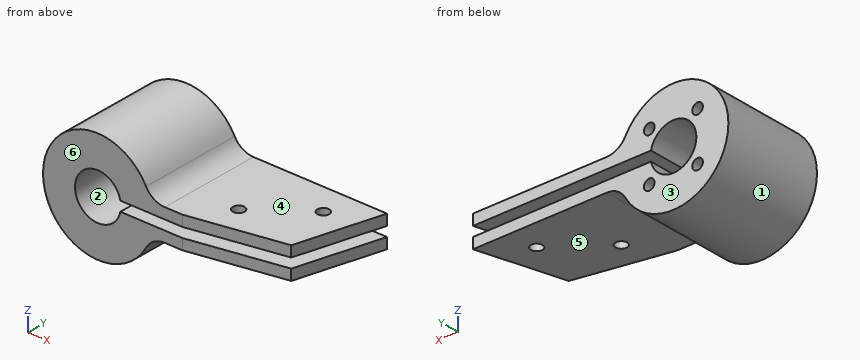
from build123d import *

# Parameters (mm, degrees)
BOSS_EXTRUDE1_DEPTH = 48
FILLET1_R           = 10
SKETCH5_R           = 2.5
CUT_EXTRUDE3_DEPTH  = 10
BOSS_EXTRUDE2_DEPTH = 5
BOSS_EXTRUDE3_DEPTH = 5
SKETCH8_R           = 2.75
CUT_EXTRUDE4_DEPTH  = 27


with BuildPart() as part:
    # Sketch1 → Boss-Extrude1 (new body)
    with BuildSketch(Plane(origin=(0, 0, 0), x_dir=(1, 0, 0), z_dir=(0, 1, 0))):
        with BuildLine():
            Line((10.511898021, 2.25), (39.708298201, 2.25))
            Line((39.708298201, 2.25), (39.708298201, 7.25))
            Line((39.708298201, 7.25), (24.708298201, 7.25))
            ThreePointArc((24.708298201, 7.25), (-25.75, 0), (24.708298201, -7.25))
            Line((24.708298201, -7.25), (39.708298201, -7.25))
            Line((39.708298201, -7.25), (39.708298201, -2.25))
            Line((39.708298201, -2.25), (10.511898021, -2.25))
            ThreePointArc((10.511898021, -2.25), (-10.75, 0), (10.511898021, 2.25))
        make_face()
    extrude(amount=BOSS_EXTRUDE1_DEPTH)

    # Fillet1
    fillet1_edges = [part.edges().sort_by_distance(p)[0] for p in [
        (24.708298201, 24, 7.25),
        (24.708298201, 24, -7.25),
    ]]
    fillet(fillet1_edges, radius=FILLET1_R)

    # Sketch5 → Cut-Extrude3 (cut)
    with BuildSketch(Plane(origin=(0, 48, 0), x_dir=(1, 0, 0), z_dir=(0, 1, 0))):
        with Locations(Location((-11.313708499, 11.313708499, 0), (0, 0, 270))):
            Circle(SKETCH5_R)
        with Locations(Location((-11.313708499, -11.313708499, 0), (0, 0, 270))):
            Circle(SKETCH5_R)
        with Locations(Location((11.313708499, -11.313708499, 0), (0, 0, 270))):
            Circle(SKETCH5_R)
        with Locations(Location((11.313708499, 11.313708499, 0), (0, 0, 270))):
            Circle(SKETCH5_R)
    extrude(amount=-CUT_EXTRUDE3_DEPTH, mode=Mode.SUBTRACT)

    # Sketch6 → Boss-Extrude2 (add)
    with BuildSketch(Plane.XY.offset(7.25)):
        Polygon((39.708298201, 0), (83.239372469, 8.461583673), (93.909140843, 48), (39.708298201, 48), align=None)
    extrude(amount=-BOSS_EXTRUDE2_DEPTH)

    # Sketch7 → Boss-Extrude3 (add)
    with BuildSketch(Plane(origin=(0, 0, -7.25), x_dir=(-1, 0, 0), z_dir=(0, 0, -1))):
        Polygon((-83.239372469, 8.461583673), (-39.708298201, 0), (-39.708298201, 48), (-93.909140843, 48), align=None)
    extrude(amount=-BOSS_EXTRUDE3_DEPTH)

    # Sketch8 → Cut-Extrude4 (cut)
    with BuildSketch(Plane(origin=(0, 0, -7.25), x_dir=(-1, 0, 0), z_dir=(0, 0, -1))):
        with Locations((-75.978050137, 34.250087132)):
            Circle(SKETCH8_R)
        with Locations((-52.123656454, 15.958069092)):
            Circle(SKETCH8_R)
    extrude(amount=-CUT_EXTRUDE4_DEPTH, mode=Mode.SUBTRACT)


solid = part.part
Verification items for the finished model (mm, model axes). Face numbers are marked on the shaded views. A direction names the side the tool comes from. Coordinates: 2 decimals unless noted, no trailing zeros. Order: outer loops, then holes, each group sorted by start corner. A loop starts at its lowest first (then second) coordinate and runs counter-clockwise, first axis right, second up.
1. Set-up check for the marked faces 4, 5 and 6: record each of +Z, -Z, +X, -X, +Y, -Y from which the full face is reachable in a straight line by a thin tool's end or side.
Results found:
face 4: +Z, +X, +Y, -Y
face 5: -Z, +X, +Y, -Y
face 6: +Z, -Z, +X, -X, -Y
2. Sectioned sample at C-C, the plane x = 76. Record the cut outline in (y, z), and give its area (3 significant figures).
Results found:
outline: (7.05, -7.25) - (31.5, -7.25) - (31.5, -2.25) - (7.05, -2.25) - close; (7.05, 2.25) - (31.5, 2.25) - (31.5, 7.25) - (7.05, 7.25) - close; (37, -7.25) - (48, -7.25) - (48, -2.25) - (37, -2.25) - close; (37, 2.25) - (48, 2.25) - (48, 7.25) - (37, 7.25) - close
area: 354 mm2
3. Sectioned sample at D-D, the plane x = 0. Record the cut outline in (y, z).
Results found:
outline: (0, -25.75) - (48, -25.75) - (48, -10.75) - (0, -10.75) - close; (0, 10.75) - (48, 10.75) - (48, 25.75) - (0, 25.75) - close
4. Release check for a two-part mould opening along X. For the marked faces 1, 2 and 3 record: +X half, -X half, draft (parallel to the pull), parting line (faces both ways), or undercut.
Results found:
face 1: parting line
face 2: undercut
face 3: draft
5. Sectioned sample at B-B, the plane y = 26.5. Record the cut outline in (x, z).
Results found:
outline: (10.51, -2.25) arc R10.75 cw (long way) to (10.51, 2.25) - (88.11, 2.25) - (88.11, 7.25) - (31.31, 7.25) arc R10 cw to (22.55, 12.42) arc R25.75 ccw (long way) to (22.55, -12.42) arc R10 cw to (31.31, -7.25) - (88.11, -7.25) - (88.11, -2.25) - close
6. Sectioned sample at A-A, the plane x = 35.5. Record the cut outline in (y, z).
Results found:
outline: (0, -7.25) - (48, -7.25) - (48, -2.25) - (0, -2.25) - close; (0, 2.25) - (48, 2.25) - (48, 7.25) - (0, 7.25) - close
7. Go/stop test with flat-tipped pins: pin 1 Ø14.5 at (x, y) = (64, 30.5) entering from -Z; pin 2 Ø1.5 at (x, z) = (-12, -11.5) entering from +Y; pin 3 Ø7 at (x, y) = (52.12, 15.96) entering from +Z; pin 4 Ø3.5 at (x, y) = (52.12, 15.96) entering from -Z. Record where each tip stops, or that it passes through.
Results found:
pin 1: stops at z = -7.25
pin 2: stops at y = 38
pin 3: stops at z = 7.25
pin 4: passes through
8. Scan lines: line 1 (Z direction, x = 42, y = 8); line 2 (Z direction, x = 0.5, y = 5.5); line 3 (Y direction, x = -13.5, z = -11.5). Record each from-to range of solid material in increasing order.
Results found:
line 1: z = -7.25 to -2.25, 2.25 to 7.25
line 2: z = -25.75 to -10.74, 10.74 to 25.75
line 3: y = 0 to 38
